Geometry check sheet. Reference: the model listing, model coordinates, mm. Face numbers are marked on the shaded views. A direction names the side the tool comes from. Round coordinates to 2 decimals unless told otherwise and drop trailing zeros. Write each loop counter-clockwise with the first axis right and the second up, starting at its lowest first coordinate (ties: lowest second). Pieces come first, ordered by that corner, then holes. Notation, with made-up numbers: M 68,16.25 L 77,16.25 A6 ccw 77,24.25 Z; hole C 62.25,-5.5 d2. An arc over 180 degrees is marked long. Use a Markdown table: item, result.
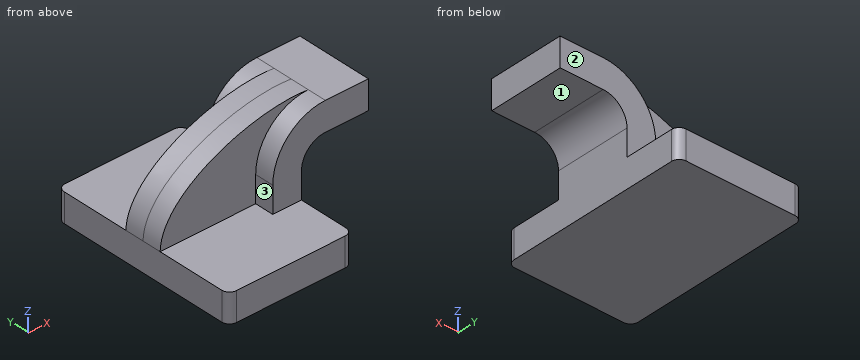
```python
from build123d import *

# Parameters (mm, degrees)
F1_DEPTH = 63.5
F0_W     = 25.4
F0_H     = 19.05
F2_DEPTH = 25.4
F3_R     = 5.08
F4_R     = 5.08
F5_R     = 5.08
F6_DEPTH = 12.7


with BuildPart() as f1:
    # F0 (on Front) → F1 (new body, symmetric)
    with BuildSketch(Plane.XZ):
        Polygon((-41.275, -9.525), (41.275, -9.525), (41.275, -1.5385041091), (41.275, 9.525), (22.225, 9.525), (-41.275, 9.525), align=None)
    extrude(amount=F1_DEPTH, both=True)

    # F0 (on Front) → F2 (join, symmetric)
    with BuildSketch(Plane.XZ):
        with BuildLine():
            Line((22.225, 9.525), (41.275, 9.525))
            Line((41.275, 9.525), (41.275, 27.0002))
            ThreePointArc((41.275, 27.0002), (45.9246798487, 38.2255201513), (57.15, 42.8752))
            Line((57.15, 42.8752), (60.325, 42.8752))
            Line((60.325, 42.8752), (60.325, 61.9252))
            Line((60.325, 61.9252), (57.15, 61.9252))
            ThreePointArc((57.15, 61.9252), (32.4542956671, 51.6959043329), (22.225, 27.0002))
            Line((22.225, 27.0002), (22.225, 9.525))
        make_face()
        with Locations((73.025, 52.4002)):
            Rectangle(F0_W, F0_H)
    extrude(amount=F2_DEPTH, both=True)

    # F3
    f3_edges = [f1.edges().sort_by_distance(p)[0] for p in [
        (-41.275, -63.5, 0),
    ]]
    fillet(f3_edges, radius=F3_R)

    # F4
    f4_edges = [f1.edges().sort_by_distance(p)[0] for p in [
        (-41.275, 63.5, 0),
        (41.275, 63.5, 0),
    ]]
    fillet(f4_edges, radius=F4_R)

    # F5
    f5_edges = [f1.edges().sort_by_distance(p)[0] for p in [
        (41.275, -63.5, 0),
    ]]
    fillet(f5_edges, radius=F5_R)

    # F0 (on Front) → F6 (join, symmetric)
    with BuildSketch(Plane.XZ):
        with BuildLine():
            add(Edge.make_bspline(
                [(-41.275, 9.525), (-40.3253436089, 42.8752), (19.9082806389, 65.561383116), (57.15, 61.9252)],
                knots=[0, 0, 0, 0, 111.5045361635, 111.5045361635, 111.5045361635, 111.5045361635], degree=3))
            Line((-41.275, 9.525), (22.225, 9.525))
            Line((22.225, 9.525), (22.225, 27.0002))
            ThreePointArc((22.225, 27.0002), (32.4542956671, 51.6959043329), (57.15, 61.9252))
        make_face()
    extrude(amount=F6_DEPTH, both=True)


solid = f1.part
```
Item 1: Cross-section at C-C, the plane x = 60. Record the cut outline in (y, z).
Outcome:
| item | result |
|---|---|
| outline | M -25.4,42.88 L 25.4,42.88 L 25.4,61.93 L -25.4,61.93 Z |
Item 2: Go/stop test with flat-tipped pins: pin 1 (18.5 mm diameter, centred on y = 18, z = 14, fed in from +X) (3 decimals); pin 2 (1 mm diameter, centred on x = 39.5, z = 49.5, fed in from -Y); pin 3 (8 mm diameter, centred on x = -16, z = 26, fed in from +Y); pin 4 (4 mm diameter, centred on x = 42, y = 44.5, fed in from -Z) (3 decimals). Record where each tip stops, or that it passes through.
Outcome:
| item | result |
|---|---|
| pin 1 | stops at x = 41.275 |
| pin 2 | stops at y = -25.4 |
| pin 3 | stops at y = 12.7 |
| pin 4 | stops at z = -9.525 |
Item 3: Cross-section at B-B, the plane y = -23. Record the cut outline in (x, z) (3 decimals), and give its area (3 significant figures).
Outcome:
| item | result |
|---|---|
| outline | M -41.275,-9.525 L 41.275,-9.525 L 41.275,27 A15.875 cw 57.15,42.875 L 85.725,42.875 L 85.725,61.925 L 57.15,61.925 A34.925 ccw 22.225,27 L 22.225,9.525 L -41.275,9.525 Z |
| area | 3,210 mm2 |
Item 4: Material ranges on line 1 along Z through (x, y) = (-27, 33.5) (3 decimals); line 2 along Y through (x, z) = (18.5, 37); line 3 along Y through (x, z) = (32, 38), recorded low to high. Write a range as from..to.
Outcome:
| item | result |
|---|---|
| line 1 | z = -9.525..9.525 |
| line 2 | y = -12.7..12.7 |
| line 3 | y = -25.4..25.4 |
Item 5: Cross-section at A-A, the plane z = 6.5. Record the cut outline in (x, y) (3 decimals), and give its area (3 significant figures).
Outcome:
| item | result |
|---|---|
| outline | M -41.275,-58.42 A5.08 ccw -36.195,-63.5 L 36.195,-63.5 A5.08 ccw 41.275,-58.42 L 41.275,58.42 A5.08 ccw 36.195,63.5 L -36.195,63.5 A5.08 ccw -41.275,58.42 Z |
| area | 10,500 mm2 |
Item 6: Cross-section at D-D, the plane y = -38. Record the cut outline in (x, z) (3 decimals).
Outcome:
| item | result |
|---|---|
| outline | M -41.275,-9.525 L 41.275,-9.525 L 41.275,9.525 L -41.275,9.525 Z |
Item 7: Access from +Z, -Z, +X, -X, +Y, -Y to the whole of each face (thin tool, end or side, straight path). Record for the marked faces 1, 2 and 3.
Outcome:
| item | result |
|---|---|
| face 1 | -Z, +X, +Y, -Y |
| face 2 | +Z, +X, -X, +Y |
| face 3 | +Z, -X, -Y |
